```python
from build123d import *


with BuildPart() as part:
    # Sweep1: sweep along a path in Sketch2
    with BuildLine(Plane(origin=(0, 0, 0), x_dir=(1, 0, 0), z_dir=(0, 1, 0))) as sweep1_path:
        Line((131.445, 11.896721187), (20.0025, 53.535245341))
        ThreePointArc((20.0025, 53.535245341), (-57.15, 0), (20.0025, -53.535245341))
        Line((20.0025, -53.535245341), (131.445, -11.896721187))
        ThreePointArc((131.445, -11.896721187), (139.7, 0), (131.445, 11.896721187))
    # Sketch3 → Sweep1 (sweep)
    with BuildSketch(Plane.XY):
        Polygon((-57.15, 3.175), (-73.025, 3.175), (-73.025, -3.175), (-57.15, -3.175), (-57.15, -0.8636), (-53.975, -0.8636), (-53.975, 0.8636), (-57.15, 0.8636), align=None)
    sweep(path=sweep1_path.line)


solid = part.part
```
Here's how the part is built. I have some questions about the finished solid (model axes, mm). A direction names the side the tool comes from. Coordinates: 2 decimals unless noted, no trailing zeros. Write each loop counter-clockwise with the first axis right and the second up, starting at its lowest first coordinate (ties: lowest second). Pieces come first, ordered by that corner, then holes. Notation, with made-up numbers: (52, 10) -> (92, 10) arc R33 ccw to (92, 44) -> close; hole circle Ø9 at (-7.75, 57). An arc over 180 degrees is marked (long way). Use a Markdown table: item, result. Add a question column.
(1) Please list where these lines run through material, in increasing order: line 1 (Z direction, x = 0, y = 0.3) (3 decimals); line 2 (Z direction, x = -2, y = 0.25); line 3 (X direction, y = -0.35, z = 0) (3 decimals).
(2) For faces 1 (the flat face through (75.39, -0.01, 29.45)), 2 (the flat face through (76.504, 2.003, 32.425)), 3 (the flat face through (82.06, 0.044, 47.295)), 4 (the flat face through (59.5, -3.175, 39.2)), 5 (the cylindrical face through (-57.13, -2, -1.54)), which set-ups out of +Z, -Z, +X, -X, +Y, -Y let a thin tool reach every point of the face, with its end or its side?
(3) If we section it at A-A, the plane x = 0: Write out the boundary of the cut face in (y, z) (3 decimals), and give its area (3 significant figures).
(4) We'd pull the mould along X, two halves only. Please class faces 6 (the flat face through (55, 3.175, -43)), 7 (the flat face through (80.5, 0.04, -47.88)), 8 (the cylindrical face through (139.7, 2, 0.2)): +X half, -X half, draft (parallel to the pull), parting line (faces both ways), or undercut.
(5) I'm going to push flat-ended pins straight in: P1, Ø2, axis at y = 0, z = -16, coming from the +X side; P2, Ø2, axis at x = 67.5, y = 2.5, coming from the +Z side. Where does each tip first touch, or does it pass through?
(6) If we section it at B-B, the plane z = 0: Write out the boundary of the cut face in (x, y) (3 decimals).
Outcome:
| question | item | result |
|---|---|---|
| 1 | line 1 | z = -73.025 to -53.975, 53.975 to 73.025 |
| 1 | line 2 | z = -73 to -53.94, 53.94 to 73 |
| 1 | line 3 | x = -73.025 to -53.975, 136.525 to 155.575 |
| 2 | face 1 | +Y, -Y |
| 2 | face 2 | +Y |
| 2 | face 3 | +Z, +X, +Y, -Y |
| 2 | face 4 | +Z, -Z, +X, -X, -Y |
| 2 | face 5 | -Y |
| 3 | outline | (-3.175, -73.025) -> (3.175, -73.025) -> (3.175, -57.15) -> (0.864, -57.15) -> (0.864, -53.975) -> (-0.864, -53.975) -> (-0.864, -57.15) -> (-3.175, -57.15) -> close; (-3.175, 57.15) -> (-0.864, 57.15) -> (-0.864, 53.975) -> (0.864, 53.975) -> (0.864, 57.15) -> (3.175, 57.15) -> (3.175, 73.025) -> (-3.175, 73.025) -> close |
| 3 | area | 213 mm^2 |
| 4 | face 6 | draft |
| 4 | face 7 | +X half |
| 4 | face 8 | undercut |
| 5 | P1 | stops at x = 151.32 |
| 5 | P2 | stops at z = 53.11 |
| 6 | outline | (-73.025, -3.175) -> (-57.15, -3.175) -> (-57.15, -0.864) -> (-53.975, -0.864) -> (-53.975, 0.864) -> (-57.15, 0.864) -> (-57.15, 3.175) -> (-73.025, 3.175) -> close; (136.525, -0.864) -> (139.7, -0.864) -> (139.7, -3.175) -> (155.575, -3.175) -> (155.575, 3.175) -> (139.7, 3.175) -> (139.7, 0.864) -> (136.525, 0.864) -> close |
